Check sheet for the drawn part. Datum: minimum x, y, z corner. Units: mm. Coordinates: 2 decimals unless noted, no trailing zeros. Write each loop counter-clockwise with the first axis right and the second up, starting at its lowest first coordinate (ties: lowest second). Pieces come first, ordered by that corner, then holes. Notation, with made-up numbers: (-30.75, -32.75) - (-25.75, -32.75) arc R36 cw to (-25.75, 4.25) - close; hole circle Ø2 at (50.5, 4.25). An arc over 180 degrees is marked (long way). Use one line per item in the form item = value. Start each with the question number.
1. Scan lines: line 1 along X through (y, z) = (24, 50); line 2 along X through (y, z) = (3.25, 50); line 3 along X through (y, z) = (19.5, 90) (1 decimal). Record each from-to range of solid material in increasing order.
2. Cross-section at A-A on y = 29.5. Give the number of separate pieces and of enclosed holes in the cut face, then the cut area to 3 significant figures.
3. Cross-section at B-B on z = 26.5. Record the boundary of the cut face in (x, y) (1 decimal).
4. Draft check along X on the marked faces 1, 2, 3 and 4. Enter one of: +X half, -X half, draft (parallel to the pull), parting line (faces both ways), or undercut.
5. Go/stop test with flat-tipped pins: pin 1 Ø4 at (x, y) = (16, 22.5) entering from +Z; pin 2 Ø3 at (x, z) = (86, 69) entering from -Y; pin 3 Ø5 at (y, z) = (26, 66) entering from +X; pin 4 Ø8 at (x, y) = (18, 29.5) entering from -Z (1 decimal). Record where each tip stops, or that it passes through.
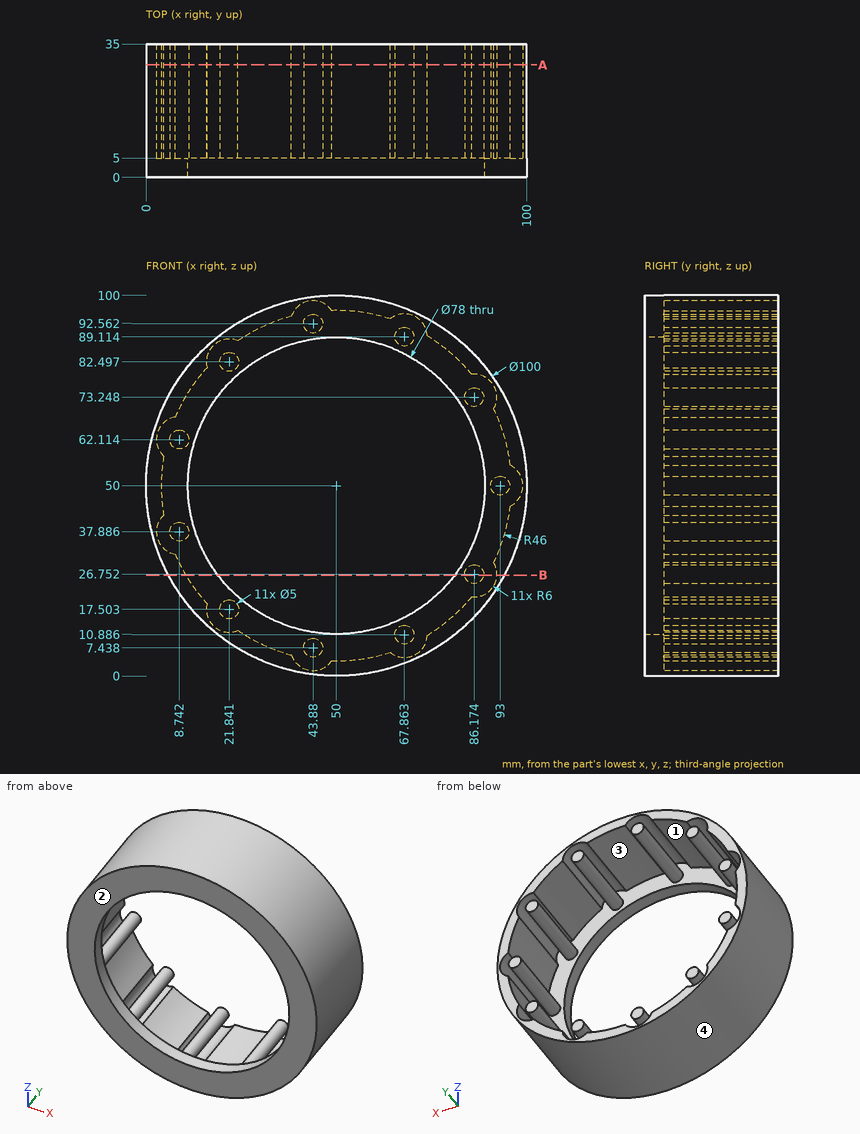
Final values:
q1.line_1 = 0 to 4, 90.5 to 95.5, 99 to 100
q1.line_2 = 0 to 11, 89 to 100
q1.line_3 = 20 to 27.3, 65.5 to 70.2, 73.8 to 80
q2.separate_pieces = 12
q2.enclosed_holes = 1
q2.area = 1,170 mm²
q3.outline = (5.9, 0) - (18.9, 0) - (18.9, 5) - (10.5, 5) - (10.5, 35) - (5.9, 35) - close; (81.1, 0) - (94.1, 0) - (94.1, 35) - (92.2, 35) - (92.2, 5) - (88.7, 5) - (88.7, 35) - (83.7, 35) - (83.7, 5) - (81.1, 5) - close
q4.face_1 = undercut
q4.face_2 = draft
q4.face_3 = undercut
q4.face_4 = parting line
q5.pin_1 = 88.42
q5.pin_2 = 0
q5.pin_3 = 98.14
q5.pin_4 = 8.6
